from build123d import *

# Parameters (mm, degrees)
SKETCH1_R           = 5
SKETCH1_R_2         = 3
BOSS_EXTRUDE1_DEPTH = 10
SKETCH2_R           = 5
SKETCH2_R_2         = 2.5
BOSS_EXTRUDE2_DEPTH = 10
SKETCH3_R           = 1.5
CUT_EXTRUDE1_DEPTH  = 10


with BuildPart() as part:
    # Sketch1 → Boss-Extrude1 (new body)
    with BuildSketch(Plane.XY):
        Circle(SKETCH1_R)
        Circle(SKETCH1_R_2, mode=Mode.SUBTRACT)
    extrude(amount=BOSS_EXTRUDE1_DEPTH)

    # Sketch2 → Boss-Extrude2 (add)
    with BuildSketch(Plane.XY.offset(10)):
        Circle(SKETCH2_R)
        Circle(SKETCH2_R_2, mode=Mode.SUBTRACT)
    extrude(amount=BOSS_EXTRUDE2_DEPTH)

    # Sketch3 → Cut-Extrude1 (cut)
    with BuildSketch(Plane(origin=(0, 0, 0), x_dir=(1, 0, 0), z_dir=(0, 1, 0))):
        with Locations((0, -5)):
            Circle(SKETCH3_R)
        with Locations((0, -15)):
            Circle(SKETCH3_R)
    extrude(amount=CUT_EXTRUDE1_DEPTH, mode=Mode.SUBTRACT)


solid = part.part
Work out the finished part from the listing and answer in its coordinate system (mm). A direction names the side the tool comes from. Round coordinates to 2 decimals unless told otherwise and drop trailing zeros. Write each loop counter-clockwise with the first axis right and the second up, starting at its lowest first coordinate (ties: lowest second). Pieces come first, ordered by that corner, then holes. Notation, with made-up numbers: (63.25, -16.5) -> (107.25, -16.5) arc R16 ccw to (107.25, -0.5) -> close; hole circle Ø3 at (40.5, 44). An arc over 180 degrees is marked (long way). Answer as CSV lines item,"result". Start each with the question number.
(1) A tool of negligible diameter and unlimited length cuts with its end or side. For faces 1 (the cylindrical face through (-0.54, -2.44, 14.93)), 2 (the flat face through (-2, 2, 10)), 3 (the cylindrical face through (-0.325, 3.785, 6.464)), from which of +Z, -Z, +X, -X, +Y, -Y can it reach the whole face along a straight path? Write none if from no direction.
(2) The part is cut by section C-C, the plane x = 1.25. Give the vertices of the cut face in (y, z), then the cut area to 3 significant figures.
(3) The part is cut by section D-D, the plane y = 4.25. Give the vertices of the cut face in (x, z).
(4) Each of these flat-tipped pins is pushed along its axis until it touches: pin 1 (2 mm diameter, centred on y = -2.5, z = 9, fed in from +X); pin 2 (1.8 mm diameter, centred on x = 1, y = 1.5, fed in from -Z). Where does it stop, or does it pass through?
(5) The part is cut by section A-A, the plane y = 0. Give the vertices of the cut face in (x, z), then the cut area to 3 significant figures.
(6) The part is cut by section B-B, the plane z = 7.75. Give the vertices of the cut face in (x, y), then the cut area to 3 significant figures.
(7) Find the intervals of material crossed by probe 1 along Z at (x, y) = (0, 4.15); probe 2 along Z at (x, y) = (0, 2.6); probe 3 along Y at (x, z) = (0, 7.25), in increasing order.
(8) The mould has two halves that part along X. Classify faces 4 (the flat face through (2, -2, 20)), 5 (the cylindrical face through (-1.08, -4.88, 9.86)), 6 (the cylindrical face through (-0.325, 3.482, 16.464)): +X half, -X half, draft (parallel to the pull), parting line (faces both ways), or undercut.
Output values:
1,face 1,"+Z, -Z"
1,face 2,"-Z"
1,face 3,"+Y"
2,outline,"(-4.84, 0) -> (-2.73, 0) -> (-2.73, 10) -> (-2.17, 10) -> (-2.17, 20) -> (-4.84, 20) -> close; (2.17, 10) -> (2.73, 10) -> (2.73, 5.83) -> (4.84, 5.83) -> (4.84, 14.17) -> (2.17, 14.17) -> close; (2.17, 15.83) -> (4.84, 15.83) -> (4.84, 20) -> (2.17, 20) -> close; (2.73, 0) -> (4.84, 0) -> (4.84, 4.17) -> (2.73, 4.17) -> close"
2,area,"87.9 mm²"
3,outline,"(-2.63, 0) -> (2.63, 0) -> (2.63, 20) -> (-2.63, 20) -> close; hole circle Ø3 at (0, 5); hole circle Ø3 at (0, 15)"
4,pin 1,"stops at x = 4.77"
4,pin 2,"stops at z = 10"
5,outline,"(-5, 0) -> (-3, 0) -> (-3, 10) -> (-2.5, 10) -> (-2.5, 20) -> (-5, 20) -> close; (2.5, 10) -> (3, 10) -> (3, 0) -> (5, 0) -> (5, 20) -> (2.5, 20) -> close"
5,area,"90.0 mm²"
6,outline,"circle Ø10 at (0, 0); hole circle Ø6 at (0, 0)"
6,area,"50.3 mm²"
7,probe 1,"z = 0 to 3.5, 6.5 to 13.5, 16.5 to 20"
7,probe 2,"z = 10 to 13.5, 16.5 to 20"
7,probe 3,"y = -5 to -3, 3 to 5"
8,face 4,"draft"
8,face 5,"parting line"
8,face 6,"undercut"
